```python
from build123d import *

# Parameters (mm, degrees)
SKETCH1_R                            = 4.7625
BOSS_EXTRUDE1_DEPTH                  = 127
F_10_32_TAPPED_HOLE1_D               = 4.0386
F_10_32_TAPPED_HOLE1_DEPTH           = 12.02944
F_10_32_TAPPED_HOLE1_TIP             = 1.213317848
F_10_32_TAPPED_HOLE1_ON_FACE_2_D     = 4.0386
F_10_32_TAPPED_HOLE1_ON_FACE_2_DEPTH = 12.02944
F_10_32_TAPPED_HOLE1_ON_FACE_2_TIP   = 1.213317848


with BuildPart() as part:
    # Sketch1 → Boss-Extrude1 (new, symmetric)
    with BuildSketch(Plane(origin=(0, 0, 0), x_dir=(0, 0, -1), z_dir=(1, 0, 0))):
        Circle(SKETCH1_R)
    extrude(amount=BOSS_EXTRUDE1_DEPTH, both=True)

    # #10-32 Tapped Hole1
    with Locations(Plane(origin=(127, 0, 0), x_dir=(0, 0, 1), z_dir=(1, 0, 0))):
        with Locations((0, 0)):
            Hole(F_10_32_TAPPED_HOLE1_D / 2, depth=F_10_32_TAPPED_HOLE1_DEPTH)
            with Locations((0, 0, -(F_10_32_TAPPED_HOLE1_DEPTH + F_10_32_TAPPED_HOLE1_TIP / 2))):  # 118° drill point
                Cone(0, F_10_32_TAPPED_HOLE1_D / 2, F_10_32_TAPPED_HOLE1_TIP, mode=Mode.SUBTRACT)

    # #10-32 Tapped Hole1 on face 2
    with Locations(Plane(origin=(-127, 0, 0), x_dir=(0, 0, -1), z_dir=(-1, 0, 0))):
        with Locations((0, 0)):
            Hole(F_10_32_TAPPED_HOLE1_ON_FACE_2_D / 2, depth=F_10_32_TAPPED_HOLE1_ON_FACE_2_DEPTH)
            with Locations((0, 0, -(F_10_32_TAPPED_HOLE1_ON_FACE_2_DEPTH + F_10_32_TAPPED_HOLE1_ON_FACE_2_TIP / 2))):  # 118° drill point
                Cone(0, F_10_32_TAPPED_HOLE1_ON_FACE_2_D / 2, F_10_32_TAPPED_HOLE1_ON_FACE_2_TIP, mode=Mode.SUBTRACT)


solid = part.part
```
Model file for the job. Use its own axes, mm. A direction names the side the tool comes from. Round coordinates to 2 decimals unless told otherwise and drop trailing zeros. Loops run counter-clockwise (first coordinate to the right, second up) from the corner with the lowest first, then second, coordinate; pieces in that order, holes last. Notation, with made-up numbers: M 39,19.25 L 57,19.25 A19 cw 57,35.25 Z; hole C 32,83 d3. An arc over 180 degrees is marked long. Put each result on its own line as item: value. Start each with the question number.
Item 1: Drill centre lines: line 1 along Y through (x, z) = (-117.5, 0); line 2 along Y through (x, z) = (-59.5, 1); line 3 along Z through (x, y) = (-10.5, 4). Where is each one in solid material? Low to high.
Item 2: 3-axis set-ups, long thin cutter, end or side, ignore diameter. For faces 4 (the face through (-127, -1, -2)), 5 (the face through (-120.901, -0.607, 1.926)), 6 (the face through (120.901, -0.607, -1.926)): which of +Z, -Z, +X, -X, +Y, -Y reach the whole face in a straight line?
Item 3: Cut at A-A (x = 96). List the corners of the cut face in (y, z) (1 decimal).
Item 4: Mould opens along Z. For faces 1 (the face through (1.78, -2.9, 3.78)), 2 (the face through (127, -1, -2)), 3 (the face through (-113.968, 0.342, 0.076)) say: released by +Z, released by -Z, zero draft, split by the parting line, or undercut.
Item 5: Drop flat-ended pins along their axis: P1, Ø1.5, axis at x = 42, y = -3, coming from the +Z side; P2, Ø5.5, axis at y = 0, z = 0, coming from the +X side; P3, Ø3, axis at x = 38.5, z = 2.5, coming from the +Y side; P4, Ø5, axis at x = -83.5, z = -3.5, coming from the -Y side. Give the stop position or say it passes through.
Answer block:
1. line 1: -4.76 to -2.02, 2.02 to 4.76
1. line 2: -4.66 to 4.66
1. line 3: -2.58 to 2.58
2. face 4: +Z, -Z, -X, +Y, -Y
2. face 5: -X
2. face 6: +X
3. outline: C 0,0 d9.5
4. face 1: split by the parting line
4. face 2: zero draft
4. face 3: undercut
5. P1: z = 4.2
5. P2: x = 127
5. P3: y = 4.66
5. P4: y = -4.66
